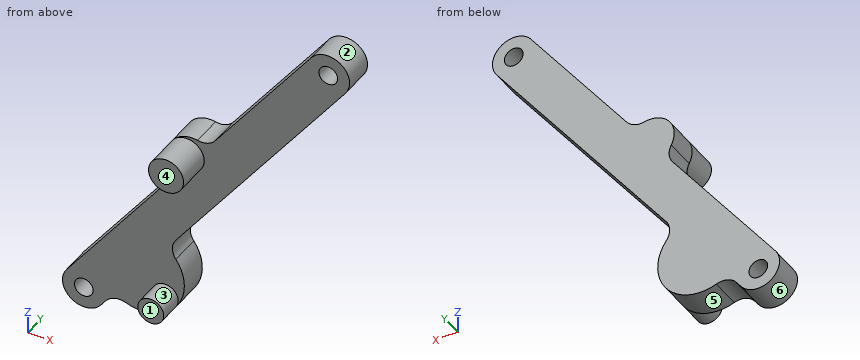
```python
from build123d import *

# Parameters (mm, degrees)
SKETCH1_R           = 1.6
BOSS_EXTRUDE1_DEPTH = 5.2
SKETCH2_R           = 3
BOSS_EXTRUDE2_DEPTH = 6
SKETCH3_R           = 2.2225
BOSS_EXTRUDE3_DEPTH = 4.21


with BuildPart() as part:
    # Sketch1 → Boss-Extrude1 (new body)
    with BuildSketch(Plane(origin=(0, 0, 0), x_dir=(1, 0, 0), z_dir=(0, 1, 0))):
        with BuildLine():
            Line((13.571690234, 65.253997386), (31.177749859, 41.779251219))
            ThreePointArc((31.177749859, 41.779251219), (31.769771696, 40.197895519), (31.413929092, 38.547273896))
            ThreePointArc((31.413929092, 38.547273896), (31.744690234, 34.020997386), (35.997302563, 32.436109267))
            ThreePointArc((35.997302563, 32.436109267), (37.681535251, 32.315544113), (39.033870608, 31.304423554))
            Line((39.033870608, 31.304423554), (55.481690234, 9.373997386))
            ThreePointArc((55.481690234, 9.373997386), (60.591690234, 8.643997386), (61.321690234, 13.753997386))
            Line((61.321690234, 13.753997386), (32.283591318, 52.471462608))
            ThreePointArc((32.283591318, 52.471462608), (31.683609832, 54.260923069), (32.271003193, 56.054555017))
            ThreePointArc((32.271003193, 56.054555017), (32.239690234, 64.967497386), (23.692033188, 67.493181691))
            ThreePointArc((23.692033188, 67.493181691), (21.805676377, 67.431501009), (20.25578915, 68.508532165))
            Line((20.25578915, 68.508532165), (19.411690234, 69.633997386))
            ThreePointArc((19.411690234, 69.633997386), (14.301690234, 70.363997386), (13.571690234, 65.253997386))
        make_face()
        with Locations(Location((16.491690234, 67.443997386, 0), (0, 0, 270))):
            Circle(SKETCH1_R, mode=Mode.SUBTRACT)
        with Locations(Location((58.401690234, 11.563997386, 0), (0, 0, 270))):
            Circle(SKETCH1_R, mode=Mode.SUBTRACT)
    extrude(amount=BOSS_EXTRUDE1_DEPTH)

    # Sketch2 → Boss-Extrude2 (add)
    with BuildSketch(Plane.XZ):
        with Locations(Location((34.144690234, -35.820997386, 0), (0, 0, 143.129227332))):
            Circle(SKETCH2_R)
    extrude(amount=BOSS_EXTRUDE2_DEPTH)

    # Sketch3 → Boss-Extrude3 (add)
    with BuildSketch(Plane.XZ):
        with Locations(Location((30.461690234, -63.633997386, 0), (0, 0, 323.129453592))):
            Circle(SKETCH3_R)
    extrude(amount=BOSS_EXTRUDE3_DEPTH)


solid = part.part
```
CAD build for the part. Positions are in the model's coordinates, mm. Face numbers are marked on the shaded views. A direction names the side the tool comes from. Round coordinates to 2 decimals unless told otherwise and drop trailing zeros. Write each loop counter-clockwise with the first axis right and the second up, starting at its lowest first coordinate (ties: lowest second). Pieces come first, ordered by that corner, then holes. Notation, with made-up numbers: (-27, 74) - (27, 74) arc R22 ccw to (27, 109) - close; hole circle Ø8 at (87, 88). An arc over 180 degrees is marked (long way). Write item = value, one per line. Start each with the question number.
Q1. Band-saw the part on B-B (y = -1.25). Give the cut face in (x, z) (1 decimal), then the cut area to 3 significant figures.
Q2. Band-saw the part on D-D (x = 26). Give the cut face in (y, z).
Q3. Mould opens along Z. For the marked faces 4, 5 and 6 say: pulls with the +Z half, pulls with the -Z half, needs draft (parallel to the pull), parting line crosses it, or undercut.
Q4. Which spindle directions (+Z, -Z, +X, -X, +Y, -Y) get a long thin tool onto all of the face, cutting with end or side? Do the marked faces 1, 2 and 3. Say none if no direction does.
Q5. Drop flat-ended pins along their axis: pin 1 (24.5 mm diameter, centred on x = 48, z = -41.5, fed in from -Y); pin 2 (4 mm diameter, centred on x = 21.5, y = 2, fed in from -Z); pin 3 (1.3 mm diameter, centred on x = 30.5, z = -63.5, fed in from -Y); pin 4 (3.5 mm diameter, centred on x = 58.4, z = -11.56, fed in from -Y). Give the stop position or say it passes through.
Q6. Band-saw the part on C-C (z = -40.5). Give the cut face in (x, y), then the cut area to 3 significant figures.
Q7. Probe L1, parallel to Y at x = 46.5, z = -31.5; L2, parallel to X at y = 3.25, z = -45; L3, parallel to Z at x = 16, y = 2. List the from-to ranges inside material, lowest first. Write a range as from..to.
Q8. Band-saw the part on A-A (y = 2.5). Count the separate pieces of the cut face and the enclosed holes in it, then the cut area to 3 significant figures.
Answers below:
q1.outline = circle Ø4.4 at (30.5, -63.6); circle Ø6 at (34.1, -35.8)
q1.area = 43.8 mm2
q2.outline = (0, -67.95) - (5.2, -67.95) - (5.2, -48.68) - (0, -48.68) - close
q3.face_4 = needs draft
q3.face_5 = undercut
q3.face_6 = parting line crosses it
q4.face_1 = -Z, +X, -X, -Y
q4.face_2 = +Y, -Y
q4.face_3 = -Y
q5.pin_1 = -6
q5.pin_2 = -69.52
q5.pin_3 = -4.21
q5.pin_4 = 0
q6.outline = (31.73, 0) - (41.26, 0) - (41.26, 5.2) - (31.73, 5.2) - close
q6.area = 49.6 mm2
q7.L1 = 0..5.2
q7.L2 = 28.76..37.89
q7.L3 = -71.06..-68.97, -65.92..-62.02
q8.separate_pieces = 1
q8.enclosed_holes = 2
q8.area = 655 mm2
